```python
from build123d import *

# Parameters (mm, degrees)
BOSS_EXTRUDE1_DEPTH = 55.88
SKETCH2_R           = 3.96875
CUT_EXTRUDE1_DEPTH  = 31.75
SKETCH3_R           = 3.175
CUT_EXTRUDE2_DEPTH  = 31.75
CUT_EXTRUDE3_DEPTH  = 91.348696172
FILLET2_R           = 6.35


with BuildPart() as part:
    # Sketch1 → Boss-Extrude1 (new body)
    with BuildSketch(Plane.XY):
        with BuildLine():
            Line((0, 0), (0, -63.5))
            Line((0, -63.5), (4.7625, -63.5))
            Line((4.7625, -63.5), (4.7625, -11.1125))
            ThreePointArc((4.7625, -11.1125), (6.622371939, -6.622371939), (11.1125, -4.7625))
            Line((11.1125, -4.7625), (31.75, -4.7625))
            Line((31.75, -4.7625), (31.75, 0))
            Line((31.75, 0), (0, 0))
        make_face()
    extrude(amount=BOSS_EXTRUDE1_DEPTH)

    # Sketch2 → Cut-Extrude1 (cut)
    with BuildSketch(Plane(origin=(0, 0, 0), x_dir=(1, 0, 0), z_dir=(0, 1, 0))):
        with Locations(Location((19.05, -27.94, 0), (0, 0, 270))):
            Circle(SKETCH2_R)
    extrude(amount=-CUT_EXTRUDE1_DEPTH, mode=Mode.SUBTRACT)

    # Sketch3 → Cut-Extrude2 (cut)
    with BuildSketch(Plane(origin=(4.7625, 0, 0), x_dir=(0, 0, -1), z_dir=(1, 0, 0))):
        with Locations((-46.355, -53.975)):
            Circle(SKETCH3_R)
        with Locations((-12.7, -53.975)):
            Circle(SKETCH3_R)
    extrude(amount=-CUT_EXTRUDE2_DEPTH, mode=Mode.SUBTRACT)

    # Sketch4 → Cut-Extrude3 (cut, through all)
    with BuildSketch(Plane(origin=(0, 0, 0), x_dir=(1, 0, 0), z_dir=(0, 1, 0))):
        Polygon((12.7, -55.88), (31.75, -36.83), (31.75, -55.88), align=None)
        Polygon((12.7, 0), (31.75, -19.05), (31.75, 0), align=None)
    extrude(amount=-CUT_EXTRUDE3_DEPTH, mode=Mode.SUBTRACT)

    # Fillet2
    fillet2_edges = [part.edges().sort_by_distance(p)[0] for p in [
        (2.38125, -63.5, 55.88),
        (31.75, -2.38125, 36.83),
        (31.75, -2.38125, 19.05),
        (2.38125, -63.5, 0),
    ]]
    fillet(fillet2_edges, radius=FILLET2_R)


solid = part.part
```
Input: part model. Units: mm. Frame: model coordinates. Coordinates: 2 decimals unless noted, no trailing zeros. Write each loop counter-clockwise with the first axis right and the second up, starting at its lowest first coordinate (ties: lowest second). Pieces come first, ordered by that corner, then holes.
1) Section A-A on z = 12.7. Output: boundary loops of the cut face in (x, y).
2) Mould query, pull axis X, two halves, no side actions, for faces 1 (the flat face through (24, -4.762, 28)), 2 (the cylindrical face through (22.4, -2.35, 30.07)), 3 (the flat face through (0, -31, 28)), 4 (the flat face through (4.762, -38, 28)). Classes: pulls with the +X half, pulls with the -X half, needs draft (parallel to the pull), parting line crosses it, or undercut.
3) Pin query (flat end, axial travel): pin 1 Ø16.5 at (x, z) = (22, 26) entering from -Y; pin 2 Ø2 at (x, z) = (19.5, 9.5) entering from +Y; pin 3 Ø12 at (x, z) = (15, 39) entering from -Y; pin 4 Ø1.5 at (x, z) = (7, 26.5) entering from -Y. Return the tip coordinate at first contact, or that it passes through.
4) Section D-D on z = 27.94. Output: boundary loops of the cut face in (x, y).
5) Section C-C on x = 4. Output: boundary loops of the cut face in (y, z) (3 decimals), and give its area (3 significant figures).
6) Section B-B on x = 19.05. Output: boundary loops of the cut face in (y, z), and give its area (3 significant figures).
7) Material intervals for line 1 along X through (y, z) = (-1.4, 27.94); line 2 along X through (y, z) = (-32.5, 52); line 3 along Y through (x, z) = (16, 52), sorted ascending.
Check result:
1. outline: (0, -63.5) - (4.76, -63.5) - (4.76, -57.15) - (0, -57.15) - close; (0, -50.8) - (4.76, -50.8) - (4.76, -11.11) arc R6.35 cw to (11.11, -4.76) - (25.4, -4.76) - (25.4, 0) - (0, 0) - close
2. face 1: needs draft
2. face 2: undercut
2. face 3: pulls with the -X half
2. face 4: pulls with the +X half
3. pin 1: stops at y = -4.76
3. pin 2: stops at y = 0
3. pin 3: stops at y = -5.12
3. pin 4: stops at y = -7.03
4. outline: (0, -63.5) - (4.76, -63.5) - (4.76, -11.11) arc R6.35 cw to (11.11, -4.76) - (15.08, -4.76) - (15.08, 0) - (0, 0) - close; (23.02, -4.76) - (31.75, -4.76) - (31.75, 0) - (23.02, 0) - close
5. outline: (-63.5, 6.35) arc R6.35 ccw to (-57.15, 0) - (0, 0) - (0, 55.88) - (-57.15, 55.88) arc R6.35 ccw to (-63.5, 49.53) - close; hole circle Ø6.35 at (-53.975, 12.7); hole circle Ø6.35 at (-53.975, 46.355)
5. area: 3,470 mm2
6. outline: (-4.76, 6.35) - (0, 6.35) - (0, 23.97) - (-4.76, 23.97) - close; (-4.76, 31.91) - (0, 31.91) - (0, 49.53) - (-4.76, 49.53) - close
6. area: 168 mm2
7. line 1: x = 0 to 15.08, 23.02 to 31.75
7. line 2: x = 0 to 4.76
7. line 3: y = -4.76 to 0
